```python
from build123d import *

# Parameters (mm, degrees)
SKETCH_1_W          = 16
SKETCH_1_H          = 12
EXTRUDE_1_DEPTH     = 7.65
SKETCH_2_W          = 5
SKETCH_2_H          = 1.2
CUT_EXTRUDE_1_DEPTH = 4.5
SKETCH_3_R          = 7.15
CUT_EXTRUDE_2_DEPTH = 1.5
SKETCH_4_W          = 16
SKETCH_4_H          = 6
EXTRUDE_2_DEPTH     = 7.5
SKETCH_5_R          = 2.25
CUT_EXTRUDE_3_DEPTH = 7.5
SKETCH_6_R          = 1.25
CUT_EXTRUDE_4_DEPTH = 8.65


with BuildPart() as part:
    # Эскиз1 → Бобышка-Вытянуть1 (new body)
    with BuildSketch(Plane.XY):
        with Locations((-13.599693696, 25)):
            Rectangle(SKETCH_1_W, SKETCH_1_H)
    extrude(amount=EXTRUDE_1_DEPTH)

    # Эскиз2 → Вырез-Вытянуть1 (cut)
    with BuildSketch(Plane.XY.offset(7.65)):
        with Locations((-19.099693696, 25)):
            Rectangle(SKETCH_2_W, SKETCH_2_H)
    extrude(amount=-CUT_EXTRUDE_1_DEPTH, mode=Mode.SUBTRACT)

    # Эскиз3 → Вырез-Вытянуть2 (cut)
    with BuildSketch(Plane.ZY.offset(16.599693696)):
        with Locations((8, 25)):
            Circle(SKETCH_3_R)
    extrude(amount=-CUT_EXTRUDE_2_DEPTH, mode=Mode.SUBTRACT)

    # Эскиз4 → Бобышка-Вытянуть2 (add)
    with BuildSketch(Plane(origin=(0, 0, 0), x_dir=(-1, 0, 0), z_dir=(0, 0, -1))):
        with Locations((13.599693696, 25)):
            Rectangle(SKETCH_4_W, SKETCH_4_H)
    extrude(amount=EXTRUDE_2_DEPTH)

    # Эскиз5 → Вырез-Вытянуть3 (cut)
    with BuildSketch(Plane(origin=(0, 0, -7.5), x_dir=(-1, 0, 0), z_dir=(0, 0, -1))):
        with Locations((10.599693696, 25)):
            Circle(SKETCH_5_R)
    extrude(amount=-CUT_EXTRUDE_3_DEPTH, mode=Mode.SUBTRACT)

    # Эскиз6 → Вырез-Вытянуть4 (cut, through all)
    with BuildSketch(Plane(origin=(0, 0, 0), x_dir=(-1, 0, 0), z_dir=(0, 0, -1))):
        with Locations((10.599693696, 25)):
            Circle(SKETCH_6_R)
    extrude(amount=-CUT_EXTRUDE_4_DEPTH, mode=Mode.SUBTRACT)


solid = part.part
```
Work out the finished part from the listing and answer in its coordinate system (mm). A direction names the side the tool comes from. Coordinates: 2 decimals unless noted, no trailing zeros. Write each loop counter-clockwise with the first axis right and the second up, starting at its lowest first coordinate (ties: lowest second). Pieces come first, ordered by that corner, then holes. Notation, with made-up numbers: (67, 71.25) - (73, 71.25) arc R33 cw to (73, 102.25) - close; hole circle Ø3 at (45, -27.75). An arc over 180 degrees is marked (long way). Answer as a JSON object with one key per item and string values.
Q1. Consider L1, parallel to Z at x = -16.75, y = 20.25; L2, parallel to Y at x = -11, z = 2.5; L3, parallel to X at y = 24, z = -5. Determine where each line is inside the solid, lowest interval first. Write a range as from..to.
Results list:
{"L1": "z = 0..7.65", "L2": "y = 19..23.82, 26.18..31", "L3": "x = -21.6..-12.62, -8.58..-5.6"}
Q2. Find section B-B (x = -8). Write down the section's boundary in (y, z).
Results list:
{"outline": "(19, 0) - (22, 0) - (22, -7.5) - (28, -7.5) - (28, 0) - (31, 0) - (31, 7.65) - (19, 7.65) - close"}
Q3. Given pin 1 Ø1.3 at (x, y) = (-10, 24.5) entering from -Z; pin 2 Ø6 at (x, z) = (-12, -5) entering from +Y; pin 3 Ø2 at (x, y) = (-10.6, 25) entering from -Z; pin 4 Ø4 at (x, y) = (-10.6, 25) entering from +Z, each flat-ended and moving along its own axis, determine where each tip first touches the part or whether it passes through.
Results list:
{"pin 1": "stops at z = 0", "pin 2": "stops at y = 28", "pin 3": "passes through", "pin 4": "stops at z = 7.65"}
Q4. Which of the six approach directions +Z, -Z, +X, -X, +Y, -Y give full straight-line access (tool end or side, diameter ignored) to faces 1 (the flat face through (-16.6, 24, 4)), 2 (the flat face through (-14, 21, 0)), 3 (the flat face through (-14, 30, 0)), 4 (the flat face through (-19, 25, 3.15))?
Results list:
{"face 1": "+Z", "face 2": "-Z, +X, -X, -Y", "face 3": "-Z, +X, -X, +Y", "face 4": "+Z, -X"}
Q5. Find section D-D (y = 22.25). Write down the section's boundary in (x, z).
Results list:
{"outline": "(-21.6, -7.5) - (-5.6, -7.5) - (-5.6, 7.65) - (-15.1, 7.65) - (-15.1, 1.4) - (-16.6, 1.4) - (-16.6, 7.65) - (-21.6, 7.65) - close"}
Q6. Find section C-C (z = 2.25). Write down the section's boundary in (x, y), plus the area to 3 significant figures.
Results list:
{"outline": "(-21.6, 19) - (-5.6, 19) - (-5.6, 31) - (-21.6, 31) - close; hole (-16.6, 20.75) - (-15.1, 20.75) - (-15.1, 29.25) - (-16.6, 29.25) - close; hole circle Ø2.5 at (-10.6, 25)", "area": "174 mm^2"}
Q7. For a pull along Y with two mould halves and no side action, classify faces 5 (the flat face through (-21.6, 25, 2)), 6 (the flat face through (-13, 22, -4)), 7 (the cylindrical face through (-15.86, 25.1, 0.85)) as pulls with the +Y half, pulls with the -Y half, needs draft (parallel to the pull), parting line crosses it, or undercut.
Results list:
{"face 5": "needs draft", "face 6": "pulls with the -Y half", "face 7": "undercut"}
Q8. Find section A-A (y = 25). Write down the section's boundary in (x, z), plus the area to 3 significant figures.
Results list:
{"outline": "(-21.6, -7.5) - (-12.85, -7.5) - (-12.85, 0) - (-11.85, 0) - (-11.85, 7.65) - (-15.1, 7.65) - (-15.1, 0.85) - (-16.6, 0.85) - (-16.6, 3.15) - (-21.6, 3.15) - close; (-9.35, 0) - (-8.35, 0) - (-8.35, -7.5) - (-5.6, -7.5) - (-5.6, 7.65) - (-9.35, 7.65) - close", "area": "157 mm^2"}
